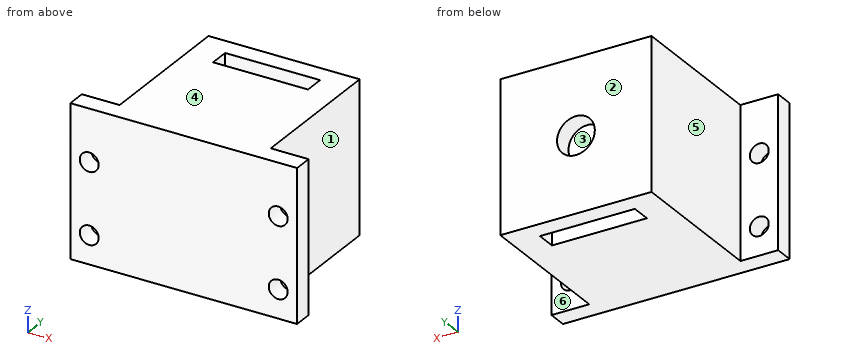
from build123d import *

# Parameters (mm, degrees)
SKETCH1_W           = 32
SKETCH1_H           = 32
BOSS_EXTRUDE1_DEPTH = 35
SKETCH2_W           = 8
SKETCH2_H           = 32
SKETCH2_R           = 2
BOSS_EXTRUDE2_DEPTH = 4
CUT_EXTRUDE1_REACH  = 55.151
SKETCH4_W           = 20.1
SKETCH4_H           = 4.2
CUT_EXTRUDE2_REACH  = 47.354
SKETCH5_R           = 4


with BuildPart() as part:
    # Sketch1 → Boss-Extrude1 (new body)
    with BuildSketch(Plane(origin=(0, 0, 0), x_dir=(1, 0, 0), z_dir=(0, 1, 0))):
        Rectangle(SKETCH1_W, SKETCH1_H)
    extrude(amount=BOSS_EXTRUDE1_DEPTH)

    # Sketch2 → Boss-Extrude2 (add)
    with BuildSketch(Plane.XZ):
        with Locations((-20, 0)):
            Rectangle(SKETCH2_W, SKETCH2_H)
        with Locations(Location((-20, 5, 0), (0, 0, 270))):
            Circle(SKETCH2_R, mode=Mode.SUBTRACT)
        with Locations(Location((-20, -10, 0), (0, 0, 270))):
            Circle(SKETCH2_R, mode=Mode.SUBTRACT)
    boss_extrude2 = extrude(amount=-BOSS_EXTRUDE2_DEPTH)

    # Mirror1: Boss-Extrude2 across plane
    add(boss_extrude2.mirror(Plane(origin=(0, 0, 0), x_dir=(0, 0, 1), z_dir=(1, 0, 0))))

    # Sketch4 → Cut-Extrude1 (cut, up to next)
    with BuildSketch(Plane(origin=(0, 0, -16), x_dir=(-1, 0, 0), z_dir=(0, 0, -1)), mode=Mode.PRIVATE) as cut_extrude1_sk1:
        with Locations((0, 28.9)):
            Rectangle(SKETCH4_W, SKETCH4_H)
    cut_extrude1_tool1 = extrude(cut_extrude1_sk1.sketch, amount=-CUT_EXTRUDE1_REACH, mode=Mode.PRIVATE) & part.part
    add(cut_extrude1_tool1.solids().sort_by_distance((0, 28.9, -16))[0], mode=Mode.SUBTRACT)

    # Sketch5 → Cut-Extrude2 (cut, up to next)
    with BuildSketch(Plane(origin=(0, 35, 0), x_dir=(1, 0, 0), z_dir=(0, 1, 0)), mode=Mode.PRIVATE) as cut_extrude2_sk1:
        with Locations(Location((0, 0, 0), (0, 0, 270))):
            Circle(SKETCH5_R)
    cut_extrude2_tool1 = extrude(cut_extrude2_sk1.sketch, amount=-CUT_EXTRUDE2_REACH, mode=Mode.PRIVATE) & part.part
    add(cut_extrude2_tool1.solids().sort_by_distance((0, 35, 0))[0], mode=Mode.SUBTRACT)


solid = part.part
Build history of the part. All positions in model axes, mm. Face numbers are marked on the shaded views. A direction names the side the tool comes from. Coordinates: 2 decimals unless noted, no trailing zeros. Order: outer loops, then holes, each group sorted by start corner. A loop starts at its lowest first (then second) coordinate and runs counter-clockwise, first axis right, second up. Notation, with made-up numbers: M -10,74 L 29,74 A27 cw 29,105 Z; hole C -33.75,38 d5. An arc over 180 degrees is marked long. One line per question, with ' | ' between items. Start each with the question number.
Q1. Saw through at B-B (x = 20). List the corners of the cut face in (y, z), then the cut area to 3 significant figures.
Q2. Probe L1, parallel to X at y = 0.8, z = -10; L2, parallel to Y at x = 8, z = 9; L3, parallel to X at y = 34, z = 0. List the from-to ranges inside material, lowest first. Write a range as from..to.
Q3. Saw through at D-D (z = -5). List the corners of the cut face in (x, y), then the cut area to 3 significant figures.
Q4. Saw through at C-C (y = 29.5). List the corners of the cut face in (x, z), then the cut area to 3 significant figures.
Q5. Two-plate mould, pull along Y, no slides. Class the marked faces 1, 2 and 3: +Y half, -Y half, draft (parallel to the pull), parting line (faces both ways), or undercut.
Q6. Saw through at A-A (z = 5). List the corners of the cut face in (x, y), then the cut area to 3 significant figures.
Q7. 3-axis set-ups, long thin cutter, end or side, ignore diameter. For the marked faces 4, 5 and 6: which of +Z, -Z, +X, -X, +Y, -Y reach the whole face in a straight line?
Q8. Flat gauge pins, fed straight in: pin 1 Ø2.5 at (x, z) = (-20, 5) entering from +Y; pin 2 Ø3.5 at (y, z) = (28.5, -0.5) entering from +X; pin 3 Ø2 at (y, z) = (28.5, -5) entering from -X; pin 4 Ø5 at (x, z) = (20, -10) entering from +Y. Where does each tip first touch, or does it go through?
Check values:
1) outline: M 0,-16 L 4,-16 L 4,-12 L 0,-12 Z; M 0,-8 L 4,-8 L 4,3 L 0,3 Z; M 0,7 L 4,7 L 4,16 L 0,16 Z | area: 96.0 mm2
2) L1: x = -24..-22, -18..18, 22..24 | L2: y = 0..26.8, 31..35 | L3: x = -16..-4, 4..16
3) outline: M -24,0 L 24,0 L 24,4 L 16,4 L 16,35 L -16,35 L -16,4 L -24,4 Z; hole M -10.05,26.8 L 10.05,26.8 L 10.05,31 L -10.05,31 Z | area: 1,100 mm2
4) outline: M -16,-16 L -10.05,-16 L -10.05,16 L -16,16 Z; M 10.05,-16 L 16,-16 L 16,16 L 10.05,16 Z | area: 381 mm2
5) face 1: draft | face 2: +Y half | face 3: undercut
6) outline: M -24,0 L -22,0 L -22,4 L -24,4 Z; M -18,0 L 18,0 L 18,4 L 16,4 L 16,35 L -16,35 L -16,4 L -18,4 Z; M 22,0 L 24,0 L 24,4 L 22,4 Z; hole M -10.05,26.8 L 10.05,26.8 L 10.05,31 L -10.05,31 Z | area: 1,070 mm2
7) face 4: +Z, +X, -X, +Y, -Y | face 5: +Z, -Z, -X, +Y | face 6: +Z, -Z, +X, +Y
8) pin 1: passes through | pin 2: stops at x = 16 | pin 3: stops at x = -16 | pin 4: stops at y = 4
